Geometry: final body of the model. Coordinates: model frame, mm. Round coordinates to 2 decimals unless told otherwise and drop trailing zeros. Write each loop counter-clockwise with the first axis right and the second up, starting at its lowest first coordinate (ties: lowest second). Pieces come first, ordered by that corner, then holes. Notation, with made-up numbers: M 35,-29.5 L 43,-29.5 A16 cw 43,-13.5 Z; hole C 24.25,4 d8. An arc over 180 degrees is marked long. Use one line per item in the form item = value. Start each with the question number.
Item 1: Section query A-A (y = 10.5). Return loops of the section in (x, z) (3 decimals), and give its area (3 significant figures).
Item 2: Ray query, probe 1 along Z at (x, y) = (24, 20); probe 2 along X at (y, z) = (0.5, 4.05); probe 3 along Y at (x, z) = (-39, 3). Return the intervals inside material, ascending.
Item 3: Section query B-B (x = 36.5). Return loops of the section in (y, z) (3 decimals).
Item 4: Section query C-C (z = 3.3). Return loops of the section in (x, y), and give its area (3 significant figures).
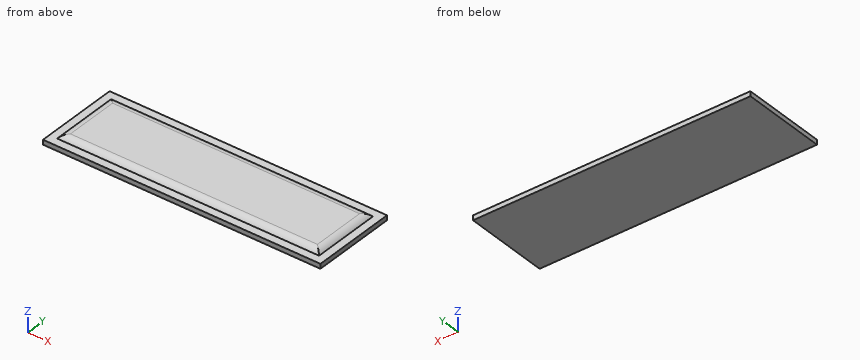
from build123d import *

# Parameters (mm, degrees)
F0_W        = 147.7690637112
F0_H        = 45.2575087547
F1_DEPTH    = 2.54
F2_W        = 139.5183503628
F2_H        = 36.5658290684
F3_DEPTH    = 1.905
F4_T1_DEPTH = 159.3462190077
F4_T3_DEPTH = 56.3936977133


# Not quite as in the source:
# - a fillet or chamfer that OpenCascade refuses, or shapes differently, is made with other operations: its cross-section is extruded or revolved along the edge and cut away or added


with BuildPart() as f1:
    # F0 (on Top) → F1 (new body)
    with BuildSketch(Plane.XY):
        Rectangle(F0_W, F0_H)
    extrude(amount=F1_DEPTH)

    # F2 (on face) → F3 (join)
    with BuildSketch(Plane.XY.offset(2.54)):
        Rectangle(F2_W, F2_H)
    extrude(amount=F3_DEPTH)

    # F4: fillet of radius 5.08 on 4 edges, made by hand

    # F4_s2 → F4_t1 (cut)
    with BuildSketch(Plane.YZ.offset(-79.6731095038)):
        with BuildLine():
            ThreePointArc((-18.2829145342, 2.54), (-16.5170453308, 3.9440501198), (-14.3173408052, 4.445))
            Line((-14.3173408052, 4.445), (-18.2829145342, 4.445))
            Line((-18.2829145342, 4.445), (-18.2829145342, 2.54))
        make_face()
        with BuildLine():
            ThreePointArc((18.2829145342, 2.54), (16.5170453308, 3.9440501198), (14.3173408052, 4.445))
            Line((14.3173408052, 4.445), (18.2829145342, 4.445))
            Line((18.2829145342, 4.445), (18.2829145342, 2.54))
        make_face()
    extrude(amount=F4_T1_DEPTH, mode=Mode.SUBTRACT)

    # F4_s4 → F4_t3 (cut)
    with BuildSketch(Plane.XZ.offset(-28.1968488567)):
        with BuildLine():
            ThreePointArc((-69.7591751814, 2.54), (-67.993305978, 3.9440501198), (-65.7936014524, 4.445))
            Line((-65.7936014524, 4.445), (-69.7591751814, 4.445))
            Line((-69.7591751814, 4.445), (-69.7591751814, 2.54))
        make_face()
        with BuildLine():
            ThreePointArc((69.7591751814, 2.54), (67.993305978, 3.9440501198), (65.7936014524, 4.445))
            Line((65.7936014524, 4.445), (69.7591751814, 4.445))
            Line((69.7591751814, 4.445), (69.7591751814, 2.54))
        make_face()
    extrude(amount=F4_T3_DEPTH, mode=Mode.SUBTRACT)


solid = f1.part
Working result:
q1.outline = M -73.885,0 L 73.885,0 L 73.885,2.54 L 69.759,2.54 A5.08 ccw 65.794,4.445 L -65.794,4.445 A5.08 ccw -69.759,2.54 L -73.885,2.54 Z
q1.area = 637 mm²
q2.probe_1 = 0 to 2.54
q2.probe_2 = -67.76 to 67.76
q2.probe_3 = -17.87 to 17.87
q3.outline = M -22.629,0 L 22.629,0 L 22.629,2.54 L 18.283,2.54 A5.08 ccw 14.317,4.445 L -14.317,4.445 A5.08 ccw -18.283,2.54 L -22.629,2.54 Z
q4.outline = M -69.01,-17.53 L 69.01,-17.53 L 69.01,17.53 L -69.01,17.53 Z
q4.area = 4,840 mm²
